Geometry check sheet. Reference: the model listing, model coordinates, mm. A direction names the side the tool comes from. Round coordinates to 2 decimals unless told otherwise and drop trailing zeros. Order: outer loops, then holes, each group sorted by start corner. A loop starts at its lowest first (then second) coordinate and runs counter-clockwise, first axis right, second up. Notation, with made-up numbers: (2.5, -13) - (14.5, -13) arc R24 cw to (14.5, 10) - close; hole circle Ø9 at (22, -29.75). An arc over 180 degrees is marked (long way). Return JSON: item names as keys, results as strings. Group by question number.
Q1. Material ranges on line 1 along Z through (x, y) = (-7, 1.25) (3 decimals); line 2 along X through (y, z) = (-0.25, 0); line 3 along Z through (x, y) = (-8, -1) (3 decimals), recorded low to high.
Q2. Sectioned sample at C-C, the plane y = 4. Record the cut outline in (x, z), then the cut area to 3 significant figures.
Q3. Sectioned sample at B-B, the plane z = -5.5. Record the cut outline in (x, y), then the cut area to 3 significant figures.
Q4. Sectioned sample at D-D, the plane x = -8. Give the number of separate pieces and of enclosed holes in the cut face, then the cut area to 3 significant figures.
Q5. Tool access check on faces 1 (the flat face through (-15, 2, -26)), 2 (the flat face through (-15, 1, -40.825)), 3 (the flat face through (-25, -1, 0)), 4 (the flat face through (-15, 1, -26.825)), 5 (the flat face through (-32, 2, 28)). Record the directions out of +Z, -Z, +X, -X, +Y, -Y that give a thin tool (end or side, any length) a straight path to the whole face; none if there is none.
Q6. Gauge pin test, flat ends, axial feed: pin 1 Ø1 at (y, z) = (-0.5, 7.5) entering from -X; pin 2 Ø0.9 at (y, z) = (1.5, -11) entering from -X; pin 3 Ø24 at (x, z) = (-16, 7.5) entering from +Y; pin 4 Ø12 at (x, z) = (-37, -25.5) entering from +Y. Record the tip position at first contact, or that the pin passes through.
Q7. Sectioned sample at A-A, the plane x = -15. Record the cut outline in (y, z) (3 decimals), then the cut area to 3 significant figures.
```python
from build123d import *

# Parameters (mm, degrees)
EXTRU_MINCE1_DEPTH      = 41
ESQUISSE2_R             = 1.5
ENL_V_MAT_EXTRU_1_DEPTH = 53.414215629
ESQUISSE3_W             = 30
ESQUISSE3_H             = 2
BOSS_EXTRU_1_DEPTH      = 2
ENL_V_MAT_EXTRU_2_DEPTH = 53.414215629
ESQUISSE5_R             = 1.2
BOSS_EXTRU_2_DEPTH      = 8.5


with BuildPart() as part:
    # Esquisse1 → Extru.-Mince1 (new, symmetric)
    with BuildSketch(Plane.XY):
        Polygon((0, 3), (0, 0), (-30, 0), (-30, 6.5), (-32, 6.5), (-32, -2), (2, -2), (2, 3), align=None)
    extrude(amount=EXTRU_MINCE1_DEPTH, both=True)

    # Esquisse2 → Enlèv. mat.-Extru.1 (cut, through all)
    with BuildSketch(Plane(origin=(0, 0, 0), x_dir=(1, 0, 0), z_dir=(0, 1, 0))):
        with Locations(Location((-8, -32.825, 0), (0, 0, 180))):
            Circle(ESQUISSE2_R)
        with Locations((-8, 32.825)):
            Circle(ESQUISSE2_R)
    extrude(amount=-ENL_V_MAT_EXTRU_1_DEPTH, mode=Mode.SUBTRACT)

    # Esquisse3 → Boss.-Extru.1 (add)
    with BuildSketch(Plane(origin=(0, 0, 0), x_dir=(1, 0, 0), z_dir=(0, 1, 0))):
        with Locations((-15, 25.825)):
            Rectangle(ESQUISSE3_W, ESQUISSE3_H)
        with Locations((-15, -25.825)):
            Rectangle(ESQUISSE3_W, ESQUISSE3_H)
        with Locations((-15, -39.825)):
            Rectangle(ESQUISSE3_W, ESQUISSE3_H)
        with Locations((-15, 39.825)):
            Rectangle(ESQUISSE3_W, ESQUISSE3_H)
    extrude(amount=BOSS_EXTRU_1_DEPTH)

    # Esquisse4 → Enlèv. mat.-Extru.2 (cut, through all)
    with BuildSketch(Plane(origin=(0, 0, 0), x_dir=(1, 0, 0), z_dir=(0, 1, 0))):
        with BuildLine():
            Line((-5, 9.825), (-5, -9.825))
            ThreePointArc((-5, -9.825), (-15, -19.825), (-25, -9.825))
            Line((-25, -9.825), (-25, 9.825))
            ThreePointArc((-25, 9.825), (-15, 19.825), (-5, 9.825))
        make_face()
    extrude(amount=-ENL_V_MAT_EXTRU_2_DEPTH, mode=Mode.SUBTRACT)

    # Esquisse5 → Boss.-Extru.2 (add)
    with BuildSketch(Plane(origin=(0, 6.5, 0), x_dir=(1, 0, 0), z_dir=(0, 1, 0))):
        with BuildLine():
            Line((-50.5, 4.330127019), (-32, 15.011106999))
            Line((-32, 15.011106999), (-32, -15.011106999))
            Line((-32, -15.011106999), (-50.5, -4.330127019))
            ThreePointArc((-50.5, -4.330127019), (-53, 0), (-50.5, 4.330127019))
        make_face()
        with Locations(Location((-48, 0, 0), (0, 0, 270))):
            Circle(ESQUISSE5_R, mode=Mode.SUBTRACT)
    extrude(amount=-BOSS_EXTRU_2_DEPTH)


solid = part.part
```
Reply:
{
 "1": {"line 1": "-40.825 to -38.825, -26.825 to -24.825, 24.825 to 26.825, 38.825 to 40.825", "line 2": "-53 to -49.2, -46.8 to -25, -5 to 2", "line 3": "-41 to -34.325, -31.325 to -16.966, 16.966 to 31.325, 34.325 to 41"},
 "2": {"outline": "(-50.5, -4.33) - (-32, -15.01) - (-32, -41) - (-30, -41) - (-30, 41) - (-32, 41) - (-32, 15.01) - (-50.5, 4.33) arc R5 ccw to start; hole circle Ø2.4 at (-48, 0)", "area": "533 mm^2"},
 "3": {"outline": "(-48.47, -2) - (-25, -2) - (-25, 0) - (-30, 0) - (-30, 6.5) - (-48.47, 6.5) - close; (-5, -2) - (2, -2) - (2, 3) - (0, 3) - (0, 0) - (-5, 0) - close", "area": "187 mm^2"},
 "4": {"separate pieces": "4", "enclosed holes": "0", "area": "100 mm^2"},
 "5": {"face 1": "+Z, -Z, +Y", "face 2": "-Z, +Y", "face 3": "+Y, -Y", "face 4": "+Y", "face 5": "+Z, -X, +Y, -Y"},
 "6": {"pin 1": "x = -45.88", "pin 2": "x = -39.73", "pin 3": "y = 0", "pin 4": "y = 6.5"},
 "7": {"outline": "(-2, -41) - (0, -41) - (0, -40.825) - (2, -40.825) - (2, -38.825) - (0, -38.825) - (0, -26.825) - (2, -26.825) - (2, -24.825) - (0, -24.825) - (0, -19.825) - (-2, -19.825) - close; (-2, 19.825) - (0, 19.825) - (0, 24.825) - (2, 24.825) - (2, 26.825) - (0, 26.825) - (0, 38.825) - (2, 38.825) - (2, 40.825) - (0, 40.825) - (0, 41) - (-2, 41) - close", "area": "101 mm^2"}
}
